```python
from build123d import *

# Parameters (mm, degrees)
SKETCH_1_R               = 10
EXTRUDE_1_DEPTH          = 63
SKETCH_2_OUTSIDE_W       = 35.812
SKETCH_2_OUTSIDE_H       = 35.812
SKETCH_2_OUTSIDE_R       = 9
CUT_EXTRUDE_1_DEPTH      = 15
SKETCH_3_R               = 6
CUT_EXTRUDE_2_DEPTH      = 65.567793829
SKETCH_4_R               = 1.5
CUT_EXTRUDE_3_DEPTH      = 65.567793829
PATTERN_CIRCULAR_1_COUNT = 2
PATTERN_CIRCULAR_1_ANGLE = 90


with BuildPart() as part:
    # 草图1 → 凸台-拉伸1 (new body)
    with BuildSketch(Plane.XY):
        Circle(SKETCH_1_R)
    extrude(amount=EXTRUDE_1_DEPTH)

    # 草图2 outside → 切除-拉伸1 (cut)
    with BuildSketch(Plane.XY.offset(63)):
        Rectangle(SKETCH_2_OUTSIDE_W, SKETCH_2_OUTSIDE_H)
        Circle(SKETCH_2_OUTSIDE_R, mode=Mode.SUBTRACT)
    extrude(amount=-CUT_EXTRUDE_1_DEPTH, mode=Mode.SUBTRACT)

    # 草图3 → 切除-拉伸2 (cut, through all)
    with BuildSketch(Plane.XY.offset(63)):
        Circle(SKETCH_3_R)
    extrude(amount=-CUT_EXTRUDE_2_DEPTH, mode=Mode.SUBTRACT)

    # 草图4 → 切除-拉伸3 (cut, symmetric)
    with BuildSketch(Plane(origin=(0, 0, 0), x_dir=(0, 0, -1), z_dir=(1, 0, 0))):
        with Locations((-26.5, 0)):
            Circle(SKETCH_4_R)
    cut_extrude_3 = extrude(amount=CUT_EXTRUDE_3_DEPTH, both=True, mode=Mode.SUBTRACT)

    # 阵列(圆周)1: 切除-拉伸3 ×2 about axis
    pattern_circular_1_axis = Axis((0, 0, 63), (0, 0, 1))
    for i in range(1, PATTERN_CIRCULAR_1_COUNT):
        add(cut_extrude_3.rotate(pattern_circular_1_axis, i * PATTERN_CIRCULAR_1_ANGLE / (PATTERN_CIRCULAR_1_COUNT - 1)), mode=Mode.SUBTRACT)


solid = part.part
```
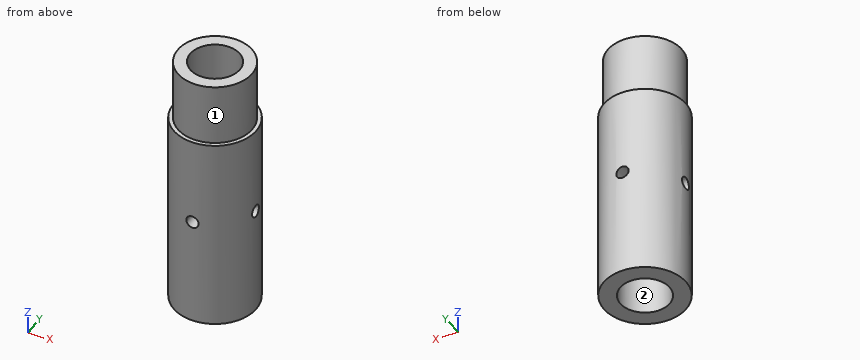
Here's how the part is built. I have some questions about the finished solid (model axes, mm). Face numbers are marked on the shaded views. A direction names the side the tool comes from. Round coordinates to 2 decimals unless told otherwise and drop trailing zeros. Order: outer loops, then holes, each group sorted by start corner. A loop starts at its lowest first (then second) coordinate and runs counter-clockwise, first axis right, second up. Notation, with made-up numbers: M 62.25,49 L 105.25,49 A17 ccw 105.25,78 Z; hole C -37,-10 d2. An arc over 180 degrees is marked long. Answer as CSV lines item,"result".
Item 1: Imagine slicing it at A-A on x = 0. List the corners of the cut face in (y, z) for me, and give its area (3 significant figures).
From the geometry:
outline,"M -10,0 L -6,0 L -6,25 L -10,25 Z; M -10,28 L -6,28 L -6,63 L -9,63 L -9,48 L -10,48 Z; M 6,0 L 10,0 L 10,25 L 6,25 Z; M 6,28 L 10,28 L 10,48 L 9,48 L 9,63 L 6,63 Z"
area,"450 mm2"
Item 2: Imagine slicing it at D-D on x = -7. List the corners of the cut face in (y, z) for me, and give its area (3 significant figures).
From the geometry:
outline,"M -7.14,0 L 7.14,0 L 7.14,48 L 5.66,48 L 5.66,63 L -5.66,63 L -5.66,48 L -7.14,48 Z; hole C 0,26.5 d3"
area,"848 mm2"
Item 3: Imagine slicing it at C-C on z = 34. List the corners of the cut face in (x, y) for me, and give its area (3 significant figures).
From the geometry:
outline,"C 0,0 d20; hole C 0,0 d12"
area,"201 mm2"
Item 4: For pin 1 (6 mm diameter, centred on x = -8, z = 56.5, fed in from -Y); pin 2 (1 mm diameter, centred on y = 6, z = 56.5, fed in from -X); pin 3 (4 mm diameter, centred on x = 6, z = 13.5, fed in from +Y), each with a flat end and sliding along its axis, tell me the tip position at first contact or that it passes through.
From the geometry:
pin 1,"y = -7.48"
pin 2,"x = -7.12"
pin 3,"y = 9.17"
Item 5: Which directions (+Z, -Z, +X, -X, +Y, -Y) give clear straight access to the entire face, cutting with the end or side of a thin tool? Please do the marked faces 1 and 2.
From the geometry:
face 1,"+Z"
face 2,"+Z, -Z"
Item 6: Imagine slicing it at B-B on z = 26.5. List the corners of the cut face in (x, y) for me, and give its area (3 significant figures).
From the geometry:
outline,"M -9.89,-1.5 A10 ccw -1.5,-9.89 L -1.5,-5.81 A6 cw -5.81,-1.5 Z; M -9.89,1.5 L -5.81,1.5 A6 cw -1.5,5.81 L -1.5,9.89 A10 ccw Z; M 1.5,-9.89 A10 ccw 9.89,-1.5 L 5.81,-1.5 A6 cw 1.5,-5.81 Z; M 1.5,5.81 A6 cw 5.81,1.5 L 9.89,1.5 A10 ccw 1.5,9.89 Z"
area,"153 mm2"
Item 7: Please list where these lines run through material, in increasing order: L1, parallel to Y at x = 0, z = 44; L2, parallel to Z at x = 0, y = -8.8. Write a range as [from, to].
From the geometry:
L1,"[-10, -6], [6, 10]"
L2,"[0, 25], [28, 63]"
